```python
from build123d import *

# Parameters (mm, degrees)
F2_DEPTH = 24.5
F0_W     = 43
F0_H     = 43
F3_DEPTH = 21.5
F5_R     = 11.1
F5_R_2   = 1.6
F6_DEPTH = 4


# Not quite as in the source:
# - a feature of the source that left no trace in its solid (it failed there, or was rolled back) is left out


with BuildPart() as f2:
    # F1 (on Right) → F2 (new body, symmetric)
    with BuildSketch(Plane.YZ):
        Polygon((21.5, 0), (-21.5, 43), (-25.5, 43), (-25.5, -4), (21.5, -4), align=None)
    extrude(amount=F2_DEPTH, both=True)

    # F0 (on Right) → F3 (cut, symmetric)
    with BuildSketch(Plane.YZ):
        with Locations((0, 21.5)):
            Rectangle(F0_W, F0_H)
    extrude(amount=F3_DEPTH, both=True, mode=Mode.SUBTRACT)

    # F5 (on face) → F6 (cut, through all)
    with BuildSketch(Plane(origin=(0, -21.5, 0), x_dir=(-1, 0, 0), z_dir=(0, 1, 0))):
        with Locations((0, 21.5)):
            Circle(F5_R)
        with Locations((15.5, 37)):
            Circle(F5_R_2)
        with Locations((-15.5, 37)):
            Circle(F5_R_2)
        with Locations((-15.5, 6)):
            Circle(F5_R_2)
        with Locations((15.5, 6)):
            Circle(F5_R_2)
    extrude(amount=-F6_DEPTH, mode=Mode.SUBTRACT)


with BuildPart() as f7:
    # F13 (on Front) → F7 (revolve)
    with BuildSketch(Plane.XZ):
        Polygon((0, -7.6705187887), (0, 0), (-3, 0), (-3, -0.5), (-1.6, -1.9), (-1.6, -7.6705187887), align=None)
    revolve(axis=Axis((0, 0, -3.8352593944), (0, 0, 1)))


with BuildPart() as f14_1:
    # F14: copy of F7
    add(f7.part.moved(Location((0, 12, 0))))


with BuildPart() as f8_1:
    # F8: copy of F7
    add(f7.part.moved(Location((0, -12, 0))))


with BuildPart() as f9_1:
    # F9: copy of F14_1
    add(f14_1.part.moved(Location((18.5, 0, 0))))


with BuildPart() as f10_1:
    # F10: instance of F9_1
    add(f9_1.part.mirror(Plane.YZ))


with BuildPart() as f15_1:
    # F15: instance of F9_1
    add(f9_1.part.mirror(Plane.XZ))


with BuildPart() as f15_2:
    # F15: instance of F10_1
    add(f10_1.part.mirror(Plane.XZ))


with BuildPart() as f2_1:
    add(f2.part)

    # F11: cut F15_1, F8_1, F15_2, F9_1, F14_1, F10_1, F7
    add(f15_1.part, mode=Mode.SUBTRACT)
    add(f8_1.part, mode=Mode.SUBTRACT)
    add(f15_2.part, mode=Mode.SUBTRACT)
    add(f9_1.part, mode=Mode.SUBTRACT)
    add(f14_1.part, mode=Mode.SUBTRACT)
    add(f10_1.part, mode=Mode.SUBTRACT)
    add(f7.part, mode=Mode.SUBTRACT)


solid = f2_1.part
```
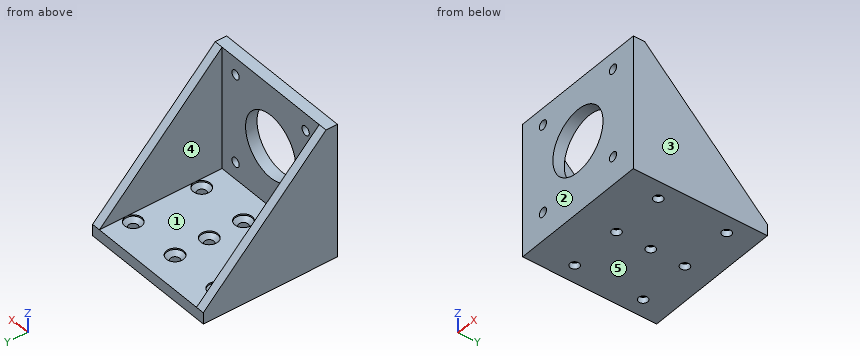
Read the model definition and answer for the solid it produces. Units are mm, in the model's axes. Face numbers are marked on the shaded views. A direction names the side the tool comes from. Round coordinates to 2 decimals unless told otherwise and drop trailing zeros. Write each loop counter-clockwise with the first axis right and the second up, starting at its lowest first coordinate (ties: lowest second). Pieces come first, ordered by that corner, then holes. Notation, with made-up numbers: (86, 76) -> (100, 76) arc R32 ccw to (100, 115) -> close; hole circle Ø10 at (-27.5, -29). An arc over 180 degrees is marked (long way). Answer in a Markdown table with one row per item. Add a question column.
1) Find section C-C, the plane y = 0. Determine the outline of the cut face in (x, z).
2) Determine the mould class of the marked faces 1, 2 and 3 for opening direction X: pulls with the +X half, pulls with the -X half, needs draft (parallel to the pull), parting line crosses it, or undercut.
3) Find section B-B, the plane z = 21.5. Determine the outline of the cut face in (x, y), and give its area (3 significant figures).
4) Consider line 1 (Y direction, x = 18.5, z = -0.3); line 2 (X direction, y = 12, z = -3.45); line 3 (X direction, y = 0, z = -0.15). Determine where each line is inside the solid, lowest interval first.
5) Find section D-D, the plane x = 0. State how many separate pieces and enclosed holes the cut face has, and give its area (3 significant figures).
6) Which of the six approach directions +Z, -Z, +X, -X, +Y, -Y give full straight-line access (tool end or side, diameter ignored) to the marked faces 4 and 5?
7) Find section A-A, the plane x = 18.5. Determine the outline of the cut face in (y, z), and give its area (3 significant figures).
8) Given P1, Ø12, axis at x = -11, z = 28.5, coming from the +Y side; P2, Ø3, axis at x = 16, y = 17, coming from the +Z side, each flat-ended and moving along its own axis, determine where each tip first touches the part or whether it passes through.
Findings below:
| question | item | result |
|---|---|---|
| 1 | outline | (-24.5, -4) -> (-1.6, -4) -> (-1.6, -1.9) -> (-3, -0.5) -> (-3, 0) -> (-21.5, 0) -> (-21.5, 21.5) -> (-24.5, 21.5) -> close; (1.6, -4) -> (24.5, -4) -> (24.5, 21.5) -> (21.5, 21.5) -> (21.5, 0) -> (3, 0) -> (3, -0.5) -> (1.6, -1.9) -> close |
| 2 | face 1 | undercut |
| 2 | face 2 | needs draft |
| 2 | face 3 | pulls with the +X half |
| 3 | outline | (-24.5, -25.5) -> (-11.1, -25.5) -> (-11.1, -21.5) -> (-21.5, -21.5) -> (-21.5, 0) -> (-24.5, 0) -> close; (11.1, -25.5) -> (24.5, -25.5) -> (24.5, 0) -> (21.5, 0) -> (21.5, -21.5) -> (11.1, -21.5) -> close |
| 3 | area | 236 mm² |
| 4 | line 1 | -25.5 to -15, -9 to 9, 15 to 21.5 |
| 4 | line 2 | -24.5 to -20.1, -16.9 to -1.6, 1.6 to 16.9, 20.1 to 24.5 |
| 4 | line 3 | -24.5 to -3, 3 to 24.5 |
| 5 | separate pieces | 5 |
| 5 | enclosed holes | 0 |
| 5 | area | 223 mm² |
| 6 | face 4 | +Z, +Y |
| 6 | face 5 | -Z, +X, -X, +Y, -Y |
| 7 | outline | (-25.5, -4) -> (-13.6, -4) -> (-13.6, -1.9) -> (-15, -0.5) -> (-15, 0) -> (-21.5, 0) -> (-21.5, 43) -> (-25.5, 43) -> close; (-10.4, -4) -> (10.4, -4) -> (10.4, -1.9) -> (9, -0.5) -> (9, 0) -> (-9, 0) -> (-9, -0.5) -> (-10.4, -1.9) -> close; (13.6, -4) -> (21.5, -4) -> (21.5, 0) -> (15, 0) -> (15, -0.5) -> (13.6, -1.9) -> close |
| 7 | area | 328 mm² |
| 8 | P1 | y = -21.5 |
| 8 | P2 | z = 0 |
